from build123d import *

# Parameters (mm, degrees)
BOSS_EXTRUDE1_START = 19.16
SKETCH1_W           = 90
SKETCH1_H           = 100
SKETCH1_R           = 2.5
SKETCH1_R_2         = 3.57
BOSS_EXTRUDE1_DEPTH = 3.18
SKETCH2_W           = 45.72
SKETCH2_H           = 65.511870912
CUT_EXTRUDE1_DEPTH  = 72.134467033
FILLET1_R           = 10
SKETCH3_R           = 2.5
CUT_EXTRUDE2_DEPTH  = 72.134467033


with BuildPart() as part:
    # Sketch1 → Boss-Extrude1 (new body)
    with BuildSketch(Plane.XY.offset(BOSS_EXTRUDE1_START)):
        with Locations((0, -5)):
            Rectangle(SKETCH1_W, SKETCH1_H)
        with Locations((32.3, -12.3)):
            Circle(SKETCH1_R, mode=Mode.SUBTRACT)
        with Locations((32.3, -42.3)):
            Circle(SKETCH1_R, mode=Mode.SUBTRACT)
        with Locations((-32.3, -42.3)):
            Circle(SKETCH1_R_2, mode=Mode.SUBTRACT)
        with Locations((-32.3, -12.3)):
            Circle(SKETCH1_R, mode=Mode.SUBTRACT)
        with Locations((-32.3, 32.3)):
            Circle(SKETCH1_R_2, mode=Mode.SUBTRACT)
        with Locations((32.3, 32.3)):
            Circle(SKETCH1_R, mode=Mode.SUBTRACT)
    extrude(amount=-BOSS_EXTRUDE1_DEPTH)

    # Sketch2 → Cut-Extrude1 (cut, through all)
    with BuildSketch(Plane(origin=(0, 0, 15.98), x_dir=(-1, 0, 0), z_dir=(0, 0, -1))):
        with Locations((0, -22.244064544)):
            Rectangle(SKETCH2_W, SKETCH2_H)
    extrude(amount=-CUT_EXTRUDE1_DEPTH, mode=Mode.SUBTRACT)

    # Fillet1
    fillet1_edges = [part.edges().sort_by_distance(p)[0] for p in [
        (22.86, 10.511870912, 17.57),
        (-22.86, 10.511870912, 17.57),
        (-45, 45, 17.57),
        (45, 45, 17.57),
        (45, -55, 17.57),
        (-45, -55, 17.57),
    ]]
    fillet(fillet1_edges, radius=FILLET1_R)

    # Sketch3 → Cut-Extrude2 (cut, through all)
    with BuildSketch(Plane.XY.offset(19.16)):
        with Locations((10, 35.930865744)):
            Circle(SKETCH3_R)
        with Locations((-10, 35.930865744)):
            Circle(SKETCH3_R)
    extrude(amount=-CUT_EXTRUDE2_DEPTH, mode=Mode.SUBTRACT)


solid = part.part
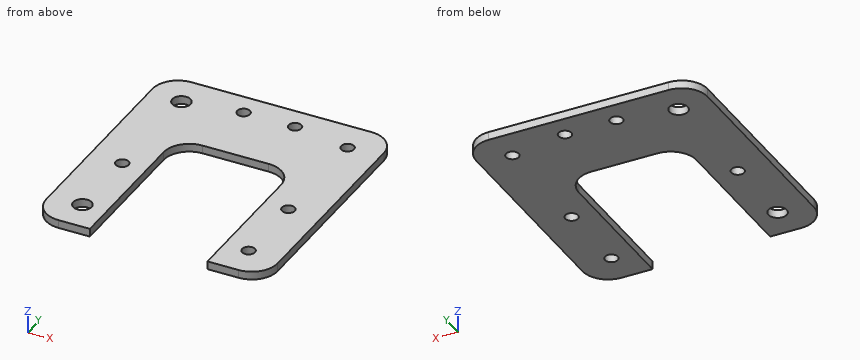
Input: part model. Units: mm. Frame: model coordinates. Round coordinates to 2 decimals unless told otherwise and drop trailing zeros. Order: outer loops, then holes, each group sorted by start corner. A loop starts at its lowest first (then second) coordinate and runs counter-clockwise, first axis right, second up. Notation, with made-up numbers: (27.25, 16.25) - (72.25, 16.25) arc R10 cw to (72.25, 29.25) - close; hole circle Ø1 at (70.5, 2.25). An arc over 180 degrees is marked (long way). Answer as a JSON object with one key per item and string values. Group by question number.
(1) Material intervals for probe 1 along Y at (x, z) = (32.3, 16.7); probe 2 along Y at (x, z) = (-32.3, 16.9); probe 3 along Y at (x, z) = (-10, 17.15), sorted ascending. Write a range as from..to.
(2) Cut plane D-D (x = -32.3). Return loops of the section in (y, z).
(3) Cut plane B-B (y = 32.3). Return loops of the section in (x, z), then the cut area to 3 significant figures.
(4) Pin query (flat end, axial travel): P1, Ø8, axis at x = -22, y = -36.5, coming from the +Z side; P2, Ø4.5, axis at x = -32.3, y = -42.3, coming from the -Z side. Return the tip coordinate at first contact, or that it passes through.
(5) Cut plane A-A (x = -10). Return loops of the section in (y, z), then the cut area to 3 significant figures.
(6) Cut plane C-C (y = -19). Return loops of the section in (x, z), then the cut area to 3 significant figures.
Here are the results:
{
 "1": {"probe 1": "y = -55..-44.8, -39.8..-14.8, -9.8..29.8, 34.8..45", "probe 2": "y = -55..-45.87, -38.73..-14.8, -9.8..28.73, 35.87..45", "probe 3": "y = 10.51..33.43, 38.43..45"},
 "2": {"outline": "(-55, 15.98) - (-45.87, 15.98) - (-45.87, 19.16) - (-55, 19.16) - close; (-38.73, 15.98) - (-14.8, 15.98) - (-14.8, 19.16) - (-38.73, 19.16) - close; (-9.8, 15.98) - (28.73, 15.98) - (28.73, 19.16) - (-9.8, 19.16) - close; (35.87, 15.98) - (45, 15.98) - (45, 19.16) - (35.87, 19.16) - close"},
 "3": {"outline": "(-45, 15.98) - (-35.87, 15.98) - (-35.87, 19.16) - (-45, 19.16) - close; (-28.73, 15.98) - (29.8, 15.98) - (29.8, 19.16) - (-28.73, 19.16) - close; (34.8, 15.98) - (45, 15.98) - (45, 19.16) - (34.8, 19.16) - close", "area": "248 mm^2"},
 "4": {"P1": "stops at z = 19.16", "P2": "passes through"},
 "5": {"outline": "(10.51, 15.98) - (33.43, 15.98) - (33.43, 19.16) - (10.51, 19.16) - close; (38.43, 15.98) - (45, 15.98) - (45, 19.16) - (38.43, 19.16) - close", "area": "93.8 mm^2"},
 "6": {"outline": "(-45, 15.98) - (-22.86, 15.98) - (-22.86, 19.16) - (-45, 19.16) - close; (22.86, 15.98) - (45, 15.98) - (45, 19.16) - (22.86, 19.16) - close", "area": "141 mm^2"}
}
